```python
from build123d import *

# Parameters (mm, degrees)
SKETCH_1_W               = 14
SKETCH_1_H               = 14
SKETCH_1_W_2             = 11.6
SKETCH_1_H_2             = 11.6
SKETCH_1_W_3             = 4.6
SKETCH_1_H_3             = 4.6
EXTRUDE_2_DEPTH          = 200
CUT_EXTRUDE_1_DEPTH      = 203.792997907
CUT_EXTRUDE_1_DEPTH_BACK = 203.792997907
SKETCH_2_R               = 2


with BuildPart() as part:
    # Эскиз1 → Бобышка-Вытянуть2 (new body)
    # profile 1 of 9: a face of its own
    with BuildSketch(Plane(origin=(0, 0, 0), x_dir=(1, 0, 0), z_dir=(0, 1, 0))):
        Polygon((8, -7), (8, -6.151471863), (6, -8.151471863), (6, -13.6), (-6, -13.6), (-6, -8.151471863), (-8, -6.151471863), (-8, -7), (-8.848528137, -7), (-7, -8.848528137), (-7, -13.4), (-8.9, -13.4), (-8.9, -12.8), (-10.9, -12.8), (-10.9, -14.2), (-10.4, -14.2), (-10.4, -15), (10.4, -15), (10.4, -14.2), (10.9, -14.2), (10.9, -12.8), (8.9, -12.8), (8.9, -13.4), (7, -13.4), (7, -8.848528137), (8.848528137, -7), align=None)
    # profile 2 of 9: a face of its own
    with BuildSketch(Plane(origin=(0, 0, 0), x_dir=(1, 0, 0), z_dir=(0, 1, 0))):
        with Locations((-15, 0)):
            Rectangle(SKETCH_1_W, SKETCH_1_H)
        with Locations((-15, 0)):
            Rectangle(SKETCH_1_W_2, SKETCH_1_H_2, mode=Mode.SUBTRACT)
    # profile 3 of 9: a face of its own
    with BuildSketch(Plane(origin=(0, 0, 0), x_dir=(1, 0, 0), z_dir=(0, 1, 0))):
        Polygon((-23, -8.848528137), (-21.151471863, -7), (-22, -7), (-22, -6.151471863), (-23.848528137, -8), (-28.4, -8), (-28.4, -6.1), (-27.8, -6.1), (-27.8, -4.1), (-29.2, -4.1), (-29.2, -4.6), (-30, -4.6), (-30, -15), (-19.6, -15), (-19.6, -14.2), (-19.1, -14.2), (-19.1, -12.8), (-21.1, -12.8), (-21.1, -13.4), (-23, -13.4), align=None)
        with Locations((-26.3, -11.3)):
            Rectangle(SKETCH_1_W_3, SKETCH_1_H_3, mode=Mode.SUBTRACT)
    # profile 4 of 9: a face of its own
    with BuildSketch(Plane(origin=(0, 0, 0), x_dir=(1, 0, 0), z_dir=(0, 1, 0))):
        with Locations((15, 0)):
            Rectangle(SKETCH_1_W, SKETCH_1_H)
        with Locations((15, 0)):
            Rectangle(SKETCH_1_W_2, SKETCH_1_H_2, mode=Mode.SUBTRACT)
    # profile 5 of 9: a face of its own
    with BuildSketch(Plane(origin=(0, 0, 0), x_dir=(1, 0, 0), z_dir=(0, 1, 0))):
        Polygon((23.848528137, -8), (22, -6.151471863), (22, -7), (21.151471863, -7), (23, -8.848528137), (23, -13.4), (21.1, -13.4), (21.1, -12.8), (19.1, -12.8), (19.1, -14.2), (19.6, -14.2), (19.6, -15), (30, -15), (30, -4.6), (29.2, -4.6), (29.2, -4.1), (27.8, -4.1), (27.8, -6.1), (28.4, -6.1), (28.4, -8), align=None)
        with Locations((26.3, -11.3)):
            Rectangle(SKETCH_1_W_3, SKETCH_1_H_3, mode=Mode.SUBTRACT)
    # profile 6 of 9: a face of its own
    with BuildSketch(Plane(origin=(0, 0, 0), x_dir=(1, 0, 0), z_dir=(0, 1, 0))):
        Polygon((21.151471863, 7), (22, 7), (22, 6.151471863), (23.848528137, 8), (28.4, 8), (28.4, 6.1), (27.8, 6.1), (27.8, 4.1), (29.2, 4.1), (29.2, 4.6), (30, 4.6), (30, 15), (19.6, 15), (19.6, 14.2), (19.1, 14.2), (19.1, 12.8), (21.1, 12.8), (21.1, 13.4), (23, 13.4), (23, 8.848528137), align=None)
        with Locations((26.3, 11.3)):
            Rectangle(SKETCH_1_W_3, SKETCH_1_H_3, mode=Mode.SUBTRACT)
    # profile 7 of 9: a face of its own
    with BuildSketch(Plane(origin=(0, 0, 0), x_dir=(1, 0, 0), z_dir=(0, 1, 0))):
        Polygon((8, 7), (8.848528137, 7), (7, 8.848528137), (7, 13.4), (8.9, 13.4), (8.9, 12.8), (10.9, 12.8), (10.9, 14.2), (10.4, 14.2), (10.4, 15), (-10.4, 15), (-10.4, 14.2), (-10.9, 14.2), (-10.9, 12.8), (-8.9, 12.8), (-8.9, 13.4), (-7, 13.4), (-7, 8.848528137), (-8.848528137, 7), (-8, 7), (-8, 6.151471863), (-6, 8.151471863), (-6, 13.6), (6, 13.6), (6, 8.151471863), (8, 6.151471863), align=None)
    # profile 8 of 9: a face of its own
    with BuildSketch(Plane(origin=(0, 0, 0), x_dir=(1, 0, 0), z_dir=(0, 1, 0))):
        Polygon((-22, 7), (-21.151471863, 7), (-23, 8.848528137), (-23, 13.4), (-21.1, 13.4), (-21.1, 12.8), (-19.1, 12.8), (-19.1, 14.2), (-19.6, 14.2), (-19.6, 15), (-30, 15), (-30, 13.6), (-28.6, 13.6), (-24, 13.6), (-24, 9), (-24, 8.151471863), (-23.848528137, 8), (-22, 6.151471863), align=None)
    # profile 9 of 9: a face of its own
    with BuildSketch(Plane(origin=(0, 0, 0), x_dir=(1, 0, 0), z_dir=(0, 1, 0))):
        Polygon((-28.6, 13.6), (-30, 13.6), (-30, 4.6), (-29.2, 4.6), (-29.2, 4.1), (-27.8, 4.1), (-27.8, 6.1), (-28.4, 6.1), (-28.4, 8), (-23.848528137, 8), (-24, 8.151471863), (-24, 9), (-28.6, 9), align=None)
    extrude(amount=EXTRUDE_2_DEPTH)

    # Эскиз2 → Вырез-Вытянуть1 (cut, two sides: drawn at the far end of the back side and taken through both)
    with BuildSketch(Plane.XY.offset(-CUT_EXTRUDE_1_DEPTH_BACK)):
        with Locations((-26, 180)):
            Circle(SKETCH_2_R)
        with Locations((-26, 80)):
            Circle(SKETCH_2_R)
    extrude(amount=CUT_EXTRUDE_1_DEPTH + CUT_EXTRUDE_1_DEPTH_BACK, mode=Mode.SUBTRACT)


solid = part.part
```
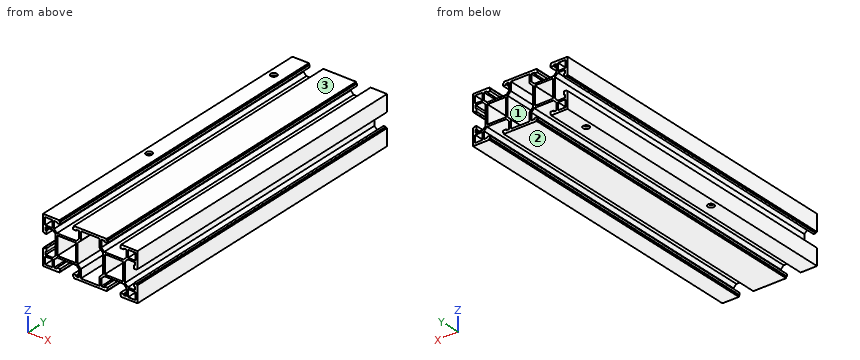
Can you work these out from the model? Positions are in its coordinate system, mm. Face numbers are marked on the shaded views. Give positions to 0.01 mm unless a question says otherwise; leave off trailing zeros. Order: outer loops, then holes, each group sorted by start corner. A loop starts at its lowest first (then second) coordinate and runs counter-clockwise, first axis right, second up. Notation, with made-up numbers: M 85,26 L 96,26 A15 cw 96,54 Z; hole C 88,15.5 d5. An arc over 180 degrees is marked long. Write item = value, one per line. Start each with the question number.
Q1. Suppose I cut it at A-A (x = 26). Write out the boundary of the cut face in (y, z).
Q2. We'd pull the mould along Z, two halves only. Please class the marked faces 1, 2 and 3: pulls with the +Z half, pulls with the -Z half, needs draft (parallel to the pull), parting line crosses it, or undercut.
Q3. I need wall thicknesses on probe 1 along X at (y, z) = (180, -14.05); probe 2 along Z at (x, y) = (20, 140); probe 3 along Y at (x, z) = (-26, 14). Which ranges of each line are inside material? Lowest first, please. Write a range as [from, to].
Q4. Suppose I cut it at C-C (y = 108). Count the separate pieces of the cut face and the enclosed holes in it, plus the area to 3 significant figures.
Q5. Suppose I cut it at B-B (x = -3.5). Write out the boundary of the cut face in (y, z), plus the area to 3 significant figures.
Q6. Will this pin go through, and if not, where does the flat tip stop? pin 1 Ø3.5 at (x, y) = (17, 80) entering from +Z.
Check result:
q1.outline = M 0,-15 L 200,-15 L 200,-13.6 L 0,-13.6 Z; M 0,-9 L 200,-9 L 200,-8 L 0,-8 Z; M 0,8 L 200,8 L 200,9 L 0,9 Z; M 0,13.6 L 200,13.6 L 200,15 L 0,15 Z
q2.face_1 = undercut
q2.face_2 = pulls with the -Z half
q2.face_3 = pulls with the +Z half
q3.probe_1 = [-30, -28], [-24, -19.1], [-10.9, 10.9], [19.1, 30]
q3.probe_2 = [-15, -12.8], [-7, -5.8], [5.8, 7], [12.8, 15]
q3.probe_3 = [0, 78], [82, 178], [182, 200]
q4.separate_pieces = 1
q4.enclosed_holes = 7
q4.area = 400 mm2
q5.outline = M 0,-15 L 200,-15 L 200,-13.6 L 0,-13.6 Z; M 0,13.6 L 200,13.6 L 200,15 L 0,15 Z
q5.area = 560 mm2
q6.pin_1 = 7
